from build123d import *

# Parameters (mm, degrees)
SKETCH2_W               = 203.2
SKETCH2_H               = 165.1
BOSS_EXTRUDE1_DEPTH     = 3.175
CUT_EXTRUDE1_REACH      = 263.836
SKETCH6_W               = 63.5
SKETCH6_H               = 63.5
CUT_EXTRUDE3_DEPTH      = 262.836457784
CUT_EXTRUDE3_DEPTH_BACK = 262.836457784
SKETCH13_R              = 19.05
SKETCH13_R_2            = 31.75
CUT_EXTRUDE4_DEPTH      = 262.836457784


with BuildPart() as part:
    # Sketch2 → Boss-Extrude1 (new body)
    with BuildSketch(Plane.XY):
        with Locations((101.6, 82.55)):
            Rectangle(SKETCH2_W, SKETCH2_H)
    extrude(amount=BOSS_EXTRUDE1_DEPTH)

    # Sketch6 → Cut-Extrude1 (cut, up to next)
    with BuildSketch(Plane(origin=(0, 0, 0), x_dir=(-1, 0, 0), z_dir=(0, 0, -1)), mode=Mode.PRIVATE) as cut_extrude1_sk1:
        with Locations((-171.45, 31.75)):
            Rectangle(SKETCH6_W, SKETCH6_H)
    cut_extrude1_tool1 = extrude(cut_extrude1_sk1.sketch, amount=-CUT_EXTRUDE1_REACH, mode=Mode.PRIVATE) & part.part
    add(cut_extrude1_tool1.solids().sort_by_distance((171.45, 31.75, 0))[0], mode=Mode.SUBTRACT)

    # Sketch7 → Cut-Extrude3 (cut, two sides: drawn at the far end of the back side and taken through both)
    with BuildSketch(Plane.XY.offset(3.175).offset(-CUT_EXTRUDE3_DEPTH_BACK)):
        Polygon((-253.570061247, 444.213374165), (165.1, 165.1), (203.2, 139.7), (621.870061247, -139.413374165), (1180.096809576, 697.926748329), (304.656687082, 1281.553496659), align=None)
    extrude(amount=CUT_EXTRUDE3_DEPTH + CUT_EXTRUDE3_DEPTH_BACK, mode=Mode.SUBTRACT)

    # Sketch13 → Cut-Extrude4 (cut, through all)
    with BuildSketch(Plane.XY.offset(3.175)):
        with Locations((127, 127)):
            Circle(SKETCH13_R)
        with Locations((63.5, 76.2)):
            Circle(SKETCH13_R_2)
    extrude(amount=-CUT_EXTRUDE4_DEPTH, mode=Mode.SUBTRACT)


solid = part.part
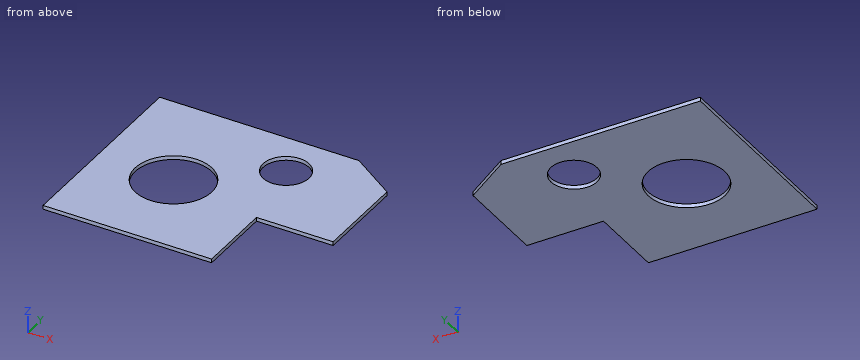
Can you work these out from the model? Positions are in its coordinate system, mm. Round coordinates to 2 decimals unless told otherwise and drop trailing zeros. Write each loop counter-clockwise with the first axis right and the second up, starting at its lowest first coordinate (ties: lowest second). Pieces come first, ordered by that corner, then holes. Notation, with made-up numbers: M 38,52.5 L 84,52.5 A31 cw 84,84.5 Z; hole C 40.5,16 d6. An arc over 180 degrees is marked long. Use a Markdown table: item, result.
Item 1: I want a section at A-A (y = 127). List the corners of the cut face in (x, z) for me (3 decimals).
Found:
| item | result |
|---|---|
| outline | M 0,0 L 107.95,0 L 107.95,3.175 L 0,3.175 Z; M 146.05,0 L 203.2,0 L 203.2,3.175 L 146.05,3.175 Z |
Item 2: I want a section at B-B (z = 0.5). List the corners of the cut face in (x, y) for me.
Found:
| item | result |
|---|---|
| outline | M 0,0 L 139.7,0 L 139.7,63.5 L 203.2,63.5 L 203.2,139.7 L 165.1,165.1 L 0,165.1 Z; hole C 63.5,76.2 d63.5; hole C 127,127 d38.1 |
Item 3: If I drill on line 1 along Y through (x, z) = (63.5, 1.8); line 2 along Y through (x, z) = (127, 1.4); line 3 along X through (y, z) = (76, 2.75), over which ranges is the centre line in solid material (lowest first)? Write a range as [from, to].
Found:
| item | result |
|---|---|
| line 1 | y = [0, 44.45], [107.95, 165.1] |
| line 2 | y = [0, 107.95], [146.05, 165.1] |
| line 3 | x = [0, 31.75], [95.25, 203.2] |
Item 4: I want a section at D-D (x = 169.5). List the corners of the cut face in (y, z) for me (3 decimals), and give its area (3 significant figures).
Found:
| item | result |
|---|---|
| outline | M 63.5,0 L 162.167,0 L 162.167,3.175 L 63.5,3.175 Z |
| area | 313 mm2 |
Item 5: I want a section at C-C (x = 63.5). List the corners of the cut face in (y, z) for me (3 decimals), and give its area (3 significant figures).
Found:
| item | result |
|---|---|
| outline | M 0,0 L 44.45,0 L 44.45,3.175 L 0,3.175 Z; M 107.95,0 L 165.1,0 L 165.1,3.175 L 107.95,3.175 Z |
| area | 323 mm2 |
Item 6: For pin 1 Ø1 at (y, z) = (23, 1) entering from +X; pin 2 Ø1 at (x, z) = (177, 1) entering from -Y, each with a flat end and sliding along its axis, tell me the tip position at first contact or that it passes through.
Found:
| item | result |
|---|---|
| pin 1 | stops at x = 139.7 |
| pin 2 | stops at y = 63.5 |
